from build123d import *

# Parameters (mm, degrees)
SKETCH1_W               = 12.7
SKETCH1_H               = 12.7
BOSS_EXTRUDE1_DEPTH     = 34.925
F_1_4_20_TAPPED_HOLE1_D = 6.35
F_1_4_20_TAPPED_HOLE2_D = 6.35
SKETCH6_W               = 12.7
SKETCH6_H               = 20.32
CUT_EXTRUDE1_DEPTH      = 13.7


with BuildPart() as part:
    # Sketch1 → Boss-Extrude1 (new body, symmetric)
    with BuildSketch(Plane.XY):
        Rectangle(SKETCH1_W, SKETCH1_H)
    extrude(amount=BOSS_EXTRUDE1_DEPTH, both=True)

    # 1/4-20 Tapped Hole1 (through all)
    with Locations(Plane(origin=(0, 6.35, 0), x_dir=(1, 0, 0), z_dir=(0, 1, 0))):
        with Locations((0, 0), (0, 19.05), (0, -19.05)):
            Hole(F_1_4_20_TAPPED_HOLE1_D / 2)

    # 1/4-20 Tapped Hole2 (through all)
    with Locations(Plane(origin=(6.35, 0, 0), x_dir=(0, 0, -1), z_dir=(1, 0, 0))):
        with Locations((9.525, 0), (28.575, 0), (-9.525, 0), (-28.575, 0)):
            Hole(F_1_4_20_TAPPED_HOLE2_D / 2)

    # Sketch6 → Cut-Extrude1 (cut, through all)
    with BuildSketch(Plane(origin=(0, 6.35, 0), x_dir=(1, 0, 0), z_dir=(0, 1, 0))):
        with Locations((0, -24.765)):
            Rectangle(SKETCH6_W, SKETCH6_H)
    extrude(amount=-CUT_EXTRUDE1_DEPTH, mode=Mode.SUBTRACT)


solid = part.part
Build history of the part. All positions in model axes, mm. Round coordinates to 2 decimals unless told otherwise and drop trailing zeros. Write each loop counter-clockwise with the first axis right and the second up, starting at its lowest first coordinate (ties: lowest second). Pieces come first, ordered by that corner, then holes. Notation, with made-up numbers: (39, 40) -> (96, 40) arc R9 cw to (96, 55) -> close; hole circle Ø10 at (22.25, 41). An arc over 180 degrees is marked (long way). Use one line per item in the form item = value.
Q1. Band-saw the part on A-A, the plane x = 0. Write the cut outline in (y, z) (3 decimals), then the cut area to 3 significant figures.
Conclusion:
outline = (-6.35, -34.925) -> (6.35, -34.925) -> (6.35, -22.225) -> (-6.35, -22.225) -> close; (-6.35, -15.875) -> (6.35, -15.875) -> (6.35, -3.175) -> (-6.35, -3.175) -> close; (-6.35, 3.175) -> (6.35, 3.175) -> (6.35, 14.605) -> (-6.35, 14.605) -> close; hole circle Ø6.35 at (0, -28.575); hole circle Ø6.35 at (0, -9.525); hole circle Ø6.35 at (0, 9.525)
area = 373 mm²
Q2. Band-saw the part on B-B, the plane y = 0. Write the cut outline in (x, z) (3 decimals).
Conclusion:
outline = (-6.35, -34.925) -> (6.35, -34.925) -> (6.35, -31.75) -> (-6.35, -31.75) -> close; (-6.35, -25.4) -> (6.35, -25.4) -> (6.35, -12.7) -> (-6.35, -12.7) -> close; (-6.35, -6.35) -> (6.35, -6.35) -> (6.35, 6.35) -> (-6.35, 6.35) -> close; (-6.35, 12.7) -> (6.35, 12.7) -> (6.35, 14.605) -> (-6.35, 14.605) -> close; hole circle Ø6.35 at (0, -19.05); hole circle Ø6.35 at (0, 0)
Q3. Band-saw the part on C-C, the plane x = -3.75. Write the cut outline in (y, z) (3 decimals), then the cut area to 3 significant figures.
Conclusion:
outline = (-6.35, -34.925) -> (6.35, -34.925) -> (6.35, 14.605) -> (-6.35, 14.605) -> close; hole circle Ø6.35 at (0, -28.575); hole circle Ø6.35 at (0, -9.525); hole circle Ø6.35 at (0, 9.525)
area = 534 mm²
Q4. Drill centre lines: L1, parallel to Z at x = 0, y = 0.25 (3 decimals); L2, parallel to Z at x = 0, y = 3.5 (3 decimals); L3, parallel to X at y = 2.75, z = -19.05 (3 decimals). Where is each one in solid material? Low to high.
Conclusion:
L1 = -34.925 to -31.74, -25.41 to -22.225, -15.875 to -12.69, -6.36 to -3.175, 3.175 to 6.36, 12.69 to 14.605
L2 = -34.925 to -22.225, -15.875 to -3.175, 3.175 to 14.605
L3 = -6.35 to -3.175, 3.175 to 6.35
Q5. Two-plate mould, pull along Z, no slides. Class faces 1 (the flat face through (0, 0, 14.605)), 2 (the flat face through (6.35, -4, -10)), 3 (the cylindrical face through (-0.089, -1.932, -12.045)): released by +Z, released by -Z, zero draft, split by the parting line, or undercut.
Conclusion:
face_1 = released by +Z
face_2 = zero draft
face_3 = undercut
Q6. Drop flat-ended pins along their axis: P1, Ø1, axis at y = 0.5, z = -26, coming from the +X side; P2, Ø5, axis at x = -1.5, z = -1.5, coming from the -Y side. Give the stop position or say it passes through.
Conclusion:
P1 = through
P2 = -6.35
Q7. Band-saw the part on D-D, the plane z = -19.05. Write the cut outline in (x, y) (3 decimals), then the cut area to 3 significant figures.
Conclusion:
outline = (-6.35, -6.35) -> (-3.175, -6.35) -> (-3.175, 6.35) -> (-6.35, 6.35) -> close; (3.175, -6.35) -> (6.35, -6.35) -> (6.35, 6.35) -> (3.175, 6.35) -> close
area = 80.6 mm²
